Input: part model. Units: mm. Frame: model coordinates. A direction names the side the tool comes from. Coordinates: 2 decimals unless noted, no trailing zeros. Loops run counter-clockwise (first coordinate to the right, second up) from the corner with the lowest first, then second, coordinate; pieces in that order, holes last. Notation, with made-up numbers: (81.5, 19.25) - (106.5, 19.25) arc R9 cw to (106.5, 23.25) - close; hole circle Ø11 at (-35.75, 75.25). An arc over 180 degrees is marked (long way). Use one line per item in the form item = value.
from build123d import *

# Parameters (mm, degrees)
EXTRUDE_1_DEPTH     = 3
SKETCH_2_W          = 5
SKETCH_2_H          = 8
CUT_EXTRUDE_1_DEPTH = 3
SKETCH_3_R          = 1.6
CUT_EXTRUDE_2_DEPTH = 3
CUT_EXTRUDE_3_REACH = 5
SKETCH_5_R          = 1.6
CUT_EXTRUDE_4_REACH = 5
SKETCH_6_R          = 0.8


with BuildPart() as part:
    # 草图1 → 凸台-拉伸1 (new body)
    with BuildSketch(Plane.XY):
        Polygon((16, 0), (-16, 0), (-16, 8), (-13, 8), (-13, 16), (-16, 16), (-16, 24), (-13, 24), (-13, 32), (-16, 32), (-16, 40), (-13, 40), (-13, 48), (-16, 48), (-16, 56), (-13, 56), (-13, 64), (13, 64), (13, 56), (16, 56), (16, 48), (13, 48), (13, 40), (16, 40), (16, 32), (13, 32), (13, 24), (16, 24), (16, 16), (13, 16), (13, 8), (16, 8), align=None)
    extrude(amount=EXTRUDE_1_DEPTH)

    # 草图2 → 切除-拉伸1 (cut)
    with BuildSketch(Plane.XY.offset(3)):
        with Locations((-4, 28)):
            Rectangle(SKETCH_2_W, SKETCH_2_H)
        with Locations((-4, 12)):
            Rectangle(SKETCH_2_W, SKETCH_2_H)
        with Locations((4, 28)):
            Rectangle(SKETCH_2_W, SKETCH_2_H)
        with Locations((-4, 44)):
            Rectangle(SKETCH_2_W, SKETCH_2_H)
        with Locations((4, 44)):
            Rectangle(SKETCH_2_W, SKETCH_2_H)
        with Locations((4, 12)):
            Rectangle(SKETCH_2_W, SKETCH_2_H)
        with Locations((4, 60)):
            Rectangle(SKETCH_2_W, SKETCH_2_H)
        with Locations((-4, 60)):
            Rectangle(SKETCH_2_W, SKETCH_2_H)
    extrude(amount=-CUT_EXTRUDE_1_DEPTH, mode=Mode.SUBTRACT)

    # 草图3 → 切除-拉伸2 (cut)
    with BuildSketch(Plane.XY.offset(3)):
        with Locations((-11.4, 4)):
            Circle(SKETCH_3_R)
        with Locations((11.4, 4)):
            Circle(SKETCH_3_R)
        with Locations((-11.4, 20)):
            Circle(SKETCH_3_R)
        with Locations((11.4, 20)):
            Circle(SKETCH_3_R)
        with Locations((-11.4, 36)):
            Circle(SKETCH_3_R)
        with Locations((11.4, 36)):
            Circle(SKETCH_3_R)
        with Locations((-11.4, 52)):
            Circle(SKETCH_3_R)
        with Locations((11.4, 52)):
            Circle(SKETCH_3_R)
    extrude(amount=-CUT_EXTRUDE_2_DEPTH, mode=Mode.SUBTRACT)

    # 草图5 → 切除-拉伸3 (cut, up to next)
    with BuildSketch(Plane.XY.offset(3), mode=Mode.PRIVATE) as cut_extrude_3_sk1:
        with Locations((-5, 4)):
            Circle(SKETCH_5_R)
    cut_extrude_3_tool1 = extrude(cut_extrude_3_sk1.sketch, amount=-CUT_EXTRUDE_3_REACH, mode=Mode.PRIVATE) & part.part
    add(cut_extrude_3_tool1.solids().sort_by_distance((-5, 4, 3))[0], mode=Mode.SUBTRACT)
    # 草图5 → 切除-拉伸3 (cut, up to next)
    with BuildSketch(Plane.XY.offset(3), mode=Mode.PRIVATE) as cut_extrude_3_sk2:
        with Locations((5, 4)):
            Circle(SKETCH_5_R)
    cut_extrude_3_tool2 = extrude(cut_extrude_3_sk2.sketch, amount=-CUT_EXTRUDE_3_REACH, mode=Mode.PRIVATE) & part.part
    add(cut_extrude_3_tool2.solids().sort_by_distance((5, 4, 3))[0], mode=Mode.SUBTRACT)
    # 草图5 → 切除-拉伸3 (cut, up to next)
    with BuildSketch(Plane.XY.offset(3), mode=Mode.PRIVATE) as cut_extrude_3_sk3:
        with Locations((-5, 20)):
            Circle(SKETCH_5_R)
    cut_extrude_3_tool3 = extrude(cut_extrude_3_sk3.sketch, amount=-CUT_EXTRUDE_3_REACH, mode=Mode.PRIVATE) & part.part
    add(cut_extrude_3_tool3.solids().sort_by_distance((-5, 20, 3))[0], mode=Mode.SUBTRACT)
    # 草图5 → 切除-拉伸3 (cut, up to next)
    with BuildSketch(Plane.XY.offset(3), mode=Mode.PRIVATE) as cut_extrude_3_sk4:
        with Locations((5, 20)):
            Circle(SKETCH_5_R)
    cut_extrude_3_tool4 = extrude(cut_extrude_3_sk4.sketch, amount=-CUT_EXTRUDE_3_REACH, mode=Mode.PRIVATE) & part.part
    add(cut_extrude_3_tool4.solids().sort_by_distance((5, 20, 3))[0], mode=Mode.SUBTRACT)
    # 草图5 → 切除-拉伸3 (cut, up to next)
    with BuildSketch(Plane.XY.offset(3), mode=Mode.PRIVATE) as cut_extrude_3_sk5:
        with Locations((-5, 36)):
            Circle(SKETCH_5_R)
    cut_extrude_3_tool5 = extrude(cut_extrude_3_sk5.sketch, amount=-CUT_EXTRUDE_3_REACH, mode=Mode.PRIVATE) & part.part
    add(cut_extrude_3_tool5.solids().sort_by_distance((-5, 36, 3))[0], mode=Mode.SUBTRACT)
    # 草图5 → 切除-拉伸3 (cut, up to next)
    with BuildSketch(Plane.XY.offset(3), mode=Mode.PRIVATE) as cut_extrude_3_sk6:
        with Locations((5, 36)):
            Circle(SKETCH_5_R)
    cut_extrude_3_tool6 = extrude(cut_extrude_3_sk6.sketch, amount=-CUT_EXTRUDE_3_REACH, mode=Mode.PRIVATE) & part.part
    add(cut_extrude_3_tool6.solids().sort_by_distance((5, 36, 3))[0], mode=Mode.SUBTRACT)
    # 草图5 → 切除-拉伸3 (cut, up to next)
    with BuildSketch(Plane.XY.offset(3), mode=Mode.PRIVATE) as cut_extrude_3_sk7:
        with Locations((-5, 52)):
            Circle(SKETCH_5_R)
    cut_extrude_3_tool7 = extrude(cut_extrude_3_sk7.sketch, amount=-CUT_EXTRUDE_3_REACH, mode=Mode.PRIVATE) & part.part
    add(cut_extrude_3_tool7.solids().sort_by_distance((-5, 52, 3))[0], mode=Mode.SUBTRACT)
    # 草图5 → 切除-拉伸3 (cut, up to next)
    with BuildSketch(Plane.XY.offset(3), mode=Mode.PRIVATE) as cut_extrude_3_sk8:
        with Locations((5, 52)):
            Circle(SKETCH_5_R)
    cut_extrude_3_tool8 = extrude(cut_extrude_3_sk8.sketch, amount=-CUT_EXTRUDE_3_REACH, mode=Mode.PRIVATE) & part.part
    add(cut_extrude_3_tool8.solids().sort_by_distance((5, 52, 3))[0], mode=Mode.SUBTRACT)

    # 草图6 → 切除-拉伸4 (cut, up to next)
    with BuildSketch(Plane.XY.offset(3), mode=Mode.PRIVATE) as cut_extrude_4_sk1:
        with Locations((-13, 8)):
            Circle(SKETCH_6_R)
    cut_extrude_4_tool1 = extrude(cut_extrude_4_sk1.sketch, amount=-CUT_EXTRUDE_4_REACH, mode=Mode.PRIVATE) & part.part
    add(cut_extrude_4_tool1.solids().sort_by_distance((-13, 8, 3))[0], mode=Mode.SUBTRACT)
    # 草图6 → 切除-拉伸4 (cut, up to next)
    with BuildSketch(Plane.XY.offset(3), mode=Mode.PRIVATE) as cut_extrude_4_sk2:
        with Locations((-13, 16)):
            Circle(SKETCH_6_R)
    cut_extrude_4_tool2 = extrude(cut_extrude_4_sk2.sketch, amount=-CUT_EXTRUDE_4_REACH, mode=Mode.PRIVATE) & part.part
    add(cut_extrude_4_tool2.solids().sort_by_distance((-13, 16, 3))[0], mode=Mode.SUBTRACT)
    # 草图6 → 切除-拉伸4 (cut, up to next)
    with BuildSketch(Plane.XY.offset(3), mode=Mode.PRIVATE) as cut_extrude_4_sk3:
        with Locations((-13, 24)):
            Circle(SKETCH_6_R)
    cut_extrude_4_tool3 = extrude(cut_extrude_4_sk3.sketch, amount=-CUT_EXTRUDE_4_REACH, mode=Mode.PRIVATE) & part.part
    add(cut_extrude_4_tool3.solids().sort_by_distance((-13, 24, 3))[0], mode=Mode.SUBTRACT)
    # 草图6 → 切除-拉伸4 (cut, up to next)
    with BuildSketch(Plane.XY.offset(3), mode=Mode.PRIVATE) as cut_extrude_4_sk4:
        with Locations((-13, 32)):
            Circle(SKETCH_6_R)
    cut_extrude_4_tool4 = extrude(cut_extrude_4_sk4.sketch, amount=-CUT_EXTRUDE_4_REACH, mode=Mode.PRIVATE) & part.part
    add(cut_extrude_4_tool4.solids().sort_by_distance((-13, 32, 3))[0], mode=Mode.SUBTRACT)
    # 草图6 → 切除-拉伸4 (cut, up to next)
    with BuildSketch(Plane.XY.offset(3), mode=Mode.PRIVATE) as cut_extrude_4_sk5:
        with Locations((-13, 40)):
            Circle(SKETCH_6_R)
    cut_extrude_4_tool5 = extrude(cut_extrude_4_sk5.sketch, amount=-CUT_EXTRUDE_4_REACH, mode=Mode.PRIVATE) & part.part
    add(cut_extrude_4_tool5.solids().sort_by_distance((-13, 40, 3))[0], mode=Mode.SUBTRACT)
    # 草图6 → 切除-拉伸4 (cut, up to next)
    with BuildSketch(Plane.XY.offset(3), mode=Mode.PRIVATE) as cut_extrude_4_sk6:
        with Locations((-13, 48)):
            Circle(SKETCH_6_R)
    cut_extrude_4_tool6 = extrude(cut_extrude_4_sk6.sketch, amount=-CUT_EXTRUDE_4_REACH, mode=Mode.PRIVATE) & part.part
    add(cut_extrude_4_tool6.solids().sort_by_distance((-13, 48, 3))[0], mode=Mode.SUBTRACT)
    # 草图6 → 切除-拉伸4 (cut, up to next)
    with BuildSketch(Plane.XY.offset(3), mode=Mode.PRIVATE) as cut_extrude_4_sk7:
        with Locations((-13, 56)):
            Circle(SKETCH_6_R)
    cut_extrude_4_tool7 = extrude(cut_extrude_4_sk7.sketch, amount=-CUT_EXTRUDE_4_REACH, mode=Mode.PRIVATE) & part.part
    add(cut_extrude_4_tool7.solids().sort_by_distance((-13, 56, 3))[0], mode=Mode.SUBTRACT)
    # 草图6 → 切除-拉伸4 (cut, up to next)
    with BuildSketch(Plane.XY.offset(3), mode=Mode.PRIVATE) as cut_extrude_4_sk8:
        with Locations((13, 8)):
            Circle(SKETCH_6_R)
    cut_extrude_4_tool8 = extrude(cut_extrude_4_sk8.sketch, amount=-CUT_EXTRUDE_4_REACH, mode=Mode.PRIVATE) & part.part
    add(cut_extrude_4_tool8.solids().sort_by_distance((13, 8, 3))[0], mode=Mode.SUBTRACT)
    # 草图6 → 切除-拉伸4 (cut, up to next)
    with BuildSketch(Plane.XY.offset(3), mode=Mode.PRIVATE) as cut_extrude_4_sk9:
        with Locations((13, 16)):
            Circle(SKETCH_6_R)
    cut_extrude_4_tool9 = extrude(cut_extrude_4_sk9.sketch, amount=-CUT_EXTRUDE_4_REACH, mode=Mode.PRIVATE) & part.part
    add(cut_extrude_4_tool9.solids().sort_by_distance((13, 16, 3))[0], mode=Mode.SUBTRACT)
    # 草图6 → 切除-拉伸4 (cut, up to next)
    with BuildSketch(Plane.XY.offset(3), mode=Mode.PRIVATE) as cut_extrude_4_sk10:
        with Locations((13, 24)):
            Circle(SKETCH_6_R)
    cut_extrude_4_tool10 = extrude(cut_extrude_4_sk10.sketch, amount=-CUT_EXTRUDE_4_REACH, mode=Mode.PRIVATE) & part.part
    add(cut_extrude_4_tool10.solids().sort_by_distance((13, 24, 3))[0], mode=Mode.SUBTRACT)
    # 草图6 → 切除-拉伸4 (cut, up to next)
    with BuildSketch(Plane.XY.offset(3), mode=Mode.PRIVATE) as cut_extrude_4_sk11:
        with Locations((13, 32)):
            Circle(SKETCH_6_R)
    cut_extrude_4_tool11 = extrude(cut_extrude_4_sk11.sketch, amount=-CUT_EXTRUDE_4_REACH, mode=Mode.PRIVATE) & part.part
    add(cut_extrude_4_tool11.solids().sort_by_distance((13, 32, 3))[0], mode=Mode.SUBTRACT)
    # 草图6 → 切除-拉伸4 (cut, up to next)
    with BuildSketch(Plane.XY.offset(3), mode=Mode.PRIVATE) as cut_extrude_4_sk12:
        with Locations((13, 40)):
            Circle(SKETCH_6_R)
    cut_extrude_4_tool12 = extrude(cut_extrude_4_sk12.sketch, amount=-CUT_EXTRUDE_4_REACH, mode=Mode.PRIVATE) & part.part
    add(cut_extrude_4_tool12.solids().sort_by_distance((13, 40, 3))[0], mode=Mode.SUBTRACT)
    # 草图6 → 切除-拉伸4 (cut, up to next)
    with BuildSketch(Plane.XY.offset(3), mode=Mode.PRIVATE) as cut_extrude_4_sk13:
        with Locations((13, 48)):
            Circle(SKETCH_6_R)
    cut_extrude_4_tool13 = extrude(cut_extrude_4_sk13.sketch, amount=-CUT_EXTRUDE_4_REACH, mode=Mode.PRIVATE) & part.part
    add(cut_extrude_4_tool13.solids().sort_by_distance((13, 48, 3))[0], mode=Mode.SUBTRACT)
    # 草图6 → 切除-拉伸4 (cut, up to next)
    with BuildSketch(Plane.XY.offset(3), mode=Mode.PRIVATE) as cut_extrude_4_sk14:
        with Locations((13, 56)):
            Circle(SKETCH_6_R)
    cut_extrude_4_tool14 = extrude(cut_extrude_4_sk14.sketch, amount=-CUT_EXTRUDE_4_REACH, mode=Mode.PRIVATE) & part.part
    add(cut_extrude_4_tool14.solids().sort_by_distance((13, 56, 3))[0], mode=Mode.SUBTRACT)


solid = part.part
Q1. Cut plane C-C, the plane x = 11.4. Return loops of the section in (y, z), then the cut area to 3 significant figures.
Check values:
outline = (0, 0) - (2.4, 0) - (2.4, 3) - (0, 3) - close; (5.6, 0) - (18.4, 0) - (18.4, 3) - (5.6, 3) - close; (21.6, 0) - (34.4, 0) - (34.4, 3) - (21.6, 3) - close; (37.6, 0) - (50.4, 0) - (50.4, 3) - (37.6, 3) - close; (53.6, 0) - (64, 0) - (64, 3) - (53.6, 3) - close
area = 154 mm²
Q2. Pull-direction query (Y, two-part tool) for faces 1 (the flat face through (16, 20, 1)), 2 (the cylindrical face through (-6.6, 52.07, 1.52)), 3 (the flat face through (-15, 56, 1)); classes: pulls with the +Y half, pulls with the -Y half, needs draft (parallel to the pull), parting line crosses it, or undercut.
Check values:
face_1 = needs draft
face_2 = undercut
face_3 = pulls with the +Y half
Q3. First-contact query: P1, Ø1.5, axis at y = 12.5, z = 1.5, coming from the -X side. Flat tip, straight axial feed; report the tip coordinate or a pass-through.
Check values:
P1 = -13
Q4. Cut plane D-D, the plane x = -5. Give the number of separate pieces and of enclosed holes in the cut face, then the cut area to 3 significant figures.
Check values:
separate_pieces = 8
enclosed_holes = 0
area = 57.6 mm²
Q5. Cut plane A-A, the plane y = 12. Return loops of the section in (x, z), then the cut area to 3 significant figures.
Check values:
outline = (-13, 0) - (-6.5, 0) - (-6.5, 3) - (-13, 3) - close; (-1.5, 0) - (1.5, 0) - (1.5, 3) - (-1.5, 3) - close; (6.5, 0) - (13, 0) - (13, 3) - (6.5, 3) - close
area = 48.0 mm²
Q6. Ray query, line 1 along X through (y, z) = (57, 0.5); line 2 along Y through (x, z) = (-11.4, 1.95); line 3 along X through (y, z) = (35, 2.45). Return the intervals inside material, ascending. Write a range as [from, to].
Check values:
line_1 = [-13, -6.5], [-1.5, 1.5], [6.5, 13]
line_2 = [0, 2.4], [5.6, 18.4], [21.6, 34.4], [37.6, 50.4], [53.6, 64]
line_3 = [-16, -12.65], [-10.15, -6.25], [-3.75, 3.75], [6.25, 10.15], [12.65, 16]
Q7. Cut plane B-B, the plane y = 52. Return loops of the section in (x, z).
Check values:
outline = (-16, 0) - (-13, 0) - (-13, 3) - (-16, 3) - close; (-9.8, 0) - (-6.6, 0) - (-6.6, 3) - (-9.8, 3) - close; (-3.4, 0) - (3.4, 0) - (3.4, 3) - (-3.4, 3) - close; (6.6, 0) - (9.8, 0) - (9.8, 3) - (6.6, 3) - close; (13, 0) - (16, 0) - (16, 3) - (13, 3) - close
Q8. Set-up query: faces 4 (the flat face through (1.5, 28, 2)), 5 (the flat face through (15, 24, 1)), 6 (the flat face through (-16, 52, 1)), 7 (the flat face through (-13, 28, 1)). Return all of +Z, -Z, +X, -X, +Y, -Y with unobstructed straight access to the full face (end or side cutting, diameter ignored); none if empty.
Check values:
face_4 = +Z, -Z
face_5 = +Z, -Z, +X
face_6 = +Z, -Z, -X, +Y, -Y
face_7 = +Z, -Z, -X
